Model file for the job. Use its own axes, mm. A direction names the side the tool comes from. Coordinates: 2 decimals unless noted, no trailing zeros. Order: outer loops, then holes, each group sorted by start corner. A loop starts at its lowest first (then second) coordinate and runs counter-clockwise, first axis right, second up. Notation, with made-up numbers: (-15.5, -33.5) -> (33.5, -33.5) arc R22 ccw to (33.5, 5.5) -> close; hole circle Ø8 at (-0.75, 79.25). An arc over 180 degrees is marked (long way). Write item = value, one per line. Start each with the question number.
Q1. Mould opens along Z. For faces 5 (the face through (116.225, 20, 48)), 6 (the face through (51, 40, 49)), 7 (the face through (-2, 62, -5)) say: +Z half, -Z half, draft (parallel to the pull), parting line (faces both ways), or undercut.
Q2. Cut at D-D, the plane x = 2. List the corners of the cut face in (y, z), plus the area to 3 significant figures.
Q3. Cut at A-A, the plane y = 62. List the corners of the cut face in (x, z) (3 decimals).
Q4. Cut at C-C, the plane y = 77. List the corners of the cut face in (x, z) (3 decimals), plus the area to 3 significant figures.
Q5. Wall check: line 1 (Z direction, x = 19.5, y = 80.5); line 2 (X direction, y = 14, z = 187.5) (3 decimals); line 3 (X direction, y = 96, z = 122.5) (3 decimals). Give the ranges that are in metal, low to high. Write a range as from..to.
Q6. Flat gauge pins, fed straight in: pin 1 (10 mm diameter, centred on x = -52.5, z = 35.5, fed in from +Y); pin 2 (10.5 mm diameter, centred on x = 86.5, z = 154.5, fed in from -Y); pin 3 (7.5 mm diameter, centred on y = 118, z = 137.5, fed in from -X) (3 decimals); pin 4 (25 mm diameter, centred on y = 77, z = 137, fed in from -X). Where does each tip first touch, or does it go through?
Q7. 3-axis set-ups, long thin cutter, end or side, ignore diameter. For faces 1 (the face through (-41.225, 20, 224)), 2 (the face through (-96.225, 91, 139)), 3 (the face through (-78, 34, 99.525)), 4 (the face through (-86.225, 115, 135)): which of +Z, -Z, +X, -X, +Y, -Y reach the whole face in a straight line?
Q8. Cut at B-B, the plane z = 72. List the corners of the cut face in (x, y) (3 decimals).
from build123d import *

# Parameters (mm, degrees)
BOSS_EXTRUDE1_DEPTH   = 274.05
BOSS_EXTRUDE1_2_DEPTH = 274.05
BOSS_EXTRUDE2_DEPTH   = 5
BOSS_EXTRUDE3_DEPTH   = 5
SKETCH4_W             = 75
SKETCH4_H             = 90
CUT_EXTRUDE4_DEPTH    = 300
SKETCH5_R             = 7.5
CUT_EXTRUDE5_DEPTH    = 10


with BuildPart() as part:
    # Sketch1 → Boss-Extrude1 (new body)
    with BuildSketch(Plane.XY):
        Polygon((-41.225, 0), (-41.225, 40), (-61.225, 40), (-61.225, 108), (-86.225, 108), (-86.225, 123), (-96.225, 123), (-96.225, 40), (-116.225, 40), (-116.225, 0), align=None)
    extrude(amount=BOSS_EXTRUDE1_DEPTH)



with BuildPart() as body_2:
    # Sketch1 → Boss-Extrude1 2 (new body)
    with BuildSketch(Plane.XY):
        Polygon((116.225, 0), (41.225, 0), (41.225, 40), (61.225, 40), (61.225, 108), (86.225, 108), (86.225, 123), (96.225, 123), (96.225, 40), (116.225, 40), align=None)
    extrude(amount=BOSS_EXTRUDE1_2_DEPTH)


with BuildPart() as part_1:
    add(part.part)

    add(body_2.part)  # Boss-Extrude2 merges body 2
    # Sketch2 → Boss-Extrude2 (add)
    with BuildSketch(Plane.XY.offset(274.05)):
        Polygon((-96.225, 123), (96.225, 123), (96.225, 40), (116.225, 40), (116.225, 0), (-116.225, 0), (-116.225, 40), (-96.225, 40), align=None)
    extrude(amount=BOSS_EXTRUDE2_DEPTH)

    # Sketch3 → Boss-Extrude3 (add)
    with BuildSketch(Plane(origin=(0, 0, 0), x_dir=(-1, 0, 0), z_dir=(0, 0, -1))):
        Polygon((-96.225, 123), (96.225, 123), (96.225, 40), (116.225, 40), (116.225, 0), (-116.225, 0), (-116.225, 40), (-96.225, 40), align=None)
    extrude(amount=BOSS_EXTRUDE3_DEPTH)

    # Sketch4 → Cut-Extrude4 (cut)
    with BuildSketch(Plane(origin=(116.225, 0, 0), x_dir=(0, 0, -1), z_dir=(1, 0, 0))):
        with Locations((-137.025, 45)):
            Rectangle(SKETCH4_W, SKETCH4_H)
    extrude(amount=-CUT_EXTRUDE4_DEPTH, mode=Mode.SUBTRACT)

    # Sketch5 → Cut-Extrude5 (cut)
    with BuildSketch(Plane.XY.offset(279.05)):
        with Locations((-49.725, 62)):
            Circle(SKETCH5_R)
        with Locations(Location((49.725, 62, 0), (0, 0, 180))):
            Circle(SKETCH5_R)
    extrude(amount=-CUT_EXTRUDE5_DEPTH, mode=Mode.SUBTRACT)


solid = part_1.part
Here are the results:
q1.face_5 = draft
q1.face_6 = undercut
q1.face_7 = -Z half
q2.outline = (0, -5) -> (123, -5) -> (123, 0) -> (0, 0) -> close; (0, 274.05) -> (123, 274.05) -> (123, 279.05) -> (0, 279.05) -> close
q2.area = 1,230 mm²
q3.outline = (-96.225, -5) -> (96.225, -5) -> (96.225, 99.525) -> (61.225, 99.525) -> (61.225, 0) -> (-61.225, 0) -> (-61.225, 99.525) -> (-96.225, 99.525) -> close; (-96.225, 174.525) -> (-61.225, 174.525) -> (-61.225, 274.05) -> (-57.225, 274.05) -> (-57.225, 279.05) -> (-96.225, 279.05) -> close; (-42.225, 274.05) -> (42.225, 274.05) -> (42.225, 279.05) -> (-42.225, 279.05) -> close; (57.225, 274.05) -> (61.225, 274.05) -> (61.225, 174.525) -> (96.225, 174.525) -> (96.225, 279.05) -> (57.225, 279.05) -> close
q4.outline = (-96.225, -5) -> (96.225, -5) -> (96.225, 99.525) -> (61.225, 99.525) -> (61.225, 0) -> (-61.225, 0) -> (-61.225, 99.525) -> (-96.225, 99.525) -> close; (-96.225, 174.525) -> (-61.225, 174.525) -> (-61.225, 274.05) -> (61.225, 274.05) -> (61.225, 174.525) -> (96.225, 174.525) -> (96.225, 279.05) -> (-96.225, 279.05) -> close
q4.area = 15,900 mm²
q5.line_1 = -5..0, 274.05..279.05
q5.line_2 = -116.225..-41.225, 41.225..116.225
q5.line_3 = -96.225..-61.225, 61.225..96.225
q6.pin_1 = 40
q6.pin_2 = 90
q6.pin_3 = -96.225
q6.pin_4 = through
q7.face_1 = +Y, -Y
q7.face_2 = +Z, -Z, -X, +Y
q7.face_3 = +X, -X, -Y
q7.face_4 = +Y
q8.outline = (-116.225, 0) -> (-41.225, 0) -> (-41.225, 40) -> (-61.225, 40) -> (-61.225, 108) -> (-86.225, 108) -> (-86.225, 123) -> (-96.225, 123) -> (-96.225, 40) -> (-116.225, 40) -> close; (41.225, 0) -> (116.225, 0) -> (116.225, 40) -> (96.225, 40) -> (96.225, 123) -> (86.225, 123) -> (86.225, 108) -> (61.225, 108) -> (61.225, 40) -> (41.225, 40) -> close
